from build123d import *

# Parameters (mm, degrees)
F1_DEPTH       = 15
F3_D           = 5
F3_CBORE_D     = 11.25
F3_CBORE_DEPTH = 6
F4_R           = 8.05
F5_DEPTH       = 2


with BuildPart() as f1:
    # F0 (on Front) → F1 (new body)
    with BuildSketch(Plane.XZ):
        Polygon((125, 0), (0, 125), (-125, 0), (0, -125), align=None)
    extrude(amount=F1_DEPTH)

    # F3 (through all)
    with Locations(Plane.XZ.offset(15)):
        with Locations((-82.5, 0), (41.25, -71.4470958122), (41.25, 71.4470958122)):
            CounterBoreHole(F3_D / 2, F3_CBORE_D / 2, F3_CBORE_DEPTH)

    # F4 (on face) → F5 (cut)
    with BuildSketch(Plane(origin=(0, 0, 0), x_dir=(-1, 0, 0), z_dir=(0, 1, 0))):
        with Locations((82.5, 0)):
            Circle(F4_R)
        with Locations((-41.25, -71.4470958122)):
            Circle(F4_R)
        with Locations((-41.25, 71.4470958122)):
            Circle(F4_R)
    extrude(amount=-F5_DEPTH, mode=Mode.SUBTRACT)


solid = f1.part
Read the model definition and answer for the solid it produces. Units are mm, in the model's axes. A direction names the side the tool comes from. Coordinates: 2 decimals unless noted, no trailing zeros. Order: outer loops, then holes, each group sorted by start corner. A loop starts at its lowest first (then second) coordinate and runs counter-clockwise, first axis right, second up. Notation, with made-up numbers: (62.25, 25) -> (119.25, 25) arc R18 ccw to (119.25, 44) -> close; hole circle Ø7 at (63.5, -34.75). An arc over 180 degrees is marked (long way). Answer as a JSON object with one key per item and string values.
1) A cutting plane is placed at A-A, the plane y = -4.5. Determine the outline of the cut face in (x, z), plus the area to 3 significant figures.
Model answer:
{"outline": "(-125, 0) -> (0, -125) -> (125, 0) -> (0, 125) -> close; hole circle Ø5 at (-82.5, 0); hole circle Ø5 at (41.25, -71.45); hole circle Ø5 at (41.25, 71.45)", "area": "31,200 mm²"}
2) A cutting plane is placed at C-C, the plane z = -88. Determine the outline of the cut face in (x, y).
Model answer:
{"outline": "(-37, -15) -> (37, -15) -> (37, 0) -> (-37, 0) -> close"}
3) Consider line 1 along Z through (x, y) = (41.25, -11.3); line 2 along Z through (x, y) = (-82.5, -6.75); line 3 along Z through (x, y) = (42.5, -9.25). Determine where each line is inside the solid, lowest interval first. Write a range as from..to.
Model answer:
{"line 1": "z = -83.75..-77.07, -65.82..65.82, 77.07..83.75", "line 2": "z = -42.5..-2.5, 2.5..42.5", "line 3": "z = -82.5..-76.93, -65.96..65.96, 76.93..82.5"}
4) A tool of negligible diameter and unlimited length cuts with its end or side. For faces 5 (the face through (63, -7, 62)), 6 (the face through (43.2, -2, 73.3)), 7 (the face through (42.4, -9, 69)), from which of +Z, -Z, +X, -X, +Y, -Y can it reach the whole face along a straight path? Write none if from no direction.
Model answer:
{"face 5": "+Z, +X, +Y, -Y", "face 6": "+Y", "face 7": "-Y"}
5) Each of these flat-tipped pins is pushed along its axis until it touches: pin 1 (13 mm diameter, centred on x = 41.25, z = -71.45, fed in from -Y); pin 2 (2 mm diameter, centred on y = -4.5, z = -15, fed in from +X); pin 3 (9 mm diameter, centred on x = -82.5, z = 0, fed in from +Y); pin 4 (8 mm diameter, centred on x = 41.25, z = -71.45, fed in from -Y). Where does it stop, or does it pass through?
Model answer:
{"pin 1": "stops at y = -15", "pin 2": "stops at x = 111", "pin 3": "stops at y = -2", "pin 4": "stops at y = -9"}
6) The mould has two halves that part along X. Classify faces 1 (the face through (-74.458, -0.986, 0.354)), 2 (the face through (-63, -7, -62)), 3 (the face through (-2, -15, 2)), 4 (the face through (-80.6, -2, 1.9)): released by +X, released by -X, zero draft, split by the parting line, or undercut.
Model answer:
{"face 1": "undercut", "face 2": "released by -X", "face 3": "zero draft", "face 4": "undercut"}
7) A cutting plane is placed at B-B, the plane x = 84.5. Determine the outline of the cut face in (y, z).
Model answer:
{"outline": "(-15, -40.5) -> (0, -40.5) -> (0, 40.5) -> (-15, 40.5) -> close"}
